```python
from build123d import *

# Parameters (mm, degrees)
RESSALTO_EXTRUS_O2_DEPTH      = 30
RESSALTO_EXTRUS_O3_START      = 3
RESSALTO_EXTRUS_O3_DEPTH      = 3
RESSALTO_EXTRUS_O4_DEPTH      = 3
RESSALTO_EXTRUS_O4_DEPTH_BACK = 10
CORTE_EXTRUS_O1_DEPTH         = 10.000000000000002
CORTE_EXTRUS_O2_REACH         = 83.702
FILETE1_R                     = 2


with BuildPart() as part:
    # Esboço2 → Ressalto-extrusão2 (new body)
    with BuildSketch(Plane(origin=(0, 0, 0), x_dir=(0, 0, -1), z_dir=(1, 0, 0))):
        with BuildLine():
            Line((2.901599919865161, -0.06246593766177921), (-35.09840008013481, -0.06246593766176534))
            Line((-35.09840008013481, -0.06246593766176534), (-39.886084902926825, -0.06246593766177921))
            ThreePointArc((-39.886084902926825, -0.06246593766177921), (-45.20218023363878, 1.4676385237390175), (-48.891439327799866, 5.589707975381692))
            ThreePointArc((-48.891439327799866, 5.589707975381692), (-52.09653694789475, 9.772081498832542), (-56.69840008013493, 12.338743680758546))
            ThreePointArc((-56.69840008013493, 12.338743680758546), (-59.37322401506481, 11.895603400997262), (-60.5984000801349, 9.476926076507686))
            Line((-60.5984000801349, 9.476926076507686), (-60.598400080134894, 20.976926076507663))
            ThreePointArc((-60.598400080134894, 20.976926076507663), (-59.71972042369454, 23.098246420067323), (-57.59840008013488, 23.976926076507684))
            Line((-57.59840008013488, 23.976926076507684), (25.401599919865156, 23.976926076507684))
            ThreePointArc((25.401599919865156, 23.976926076507684), (27.522920263424812, 23.098246420067333), (28.401599919865177, 20.976926076507684))
            Line((28.401599919865177, 20.976926076507684), (28.40159991986526, 9.476926076507686))
            ThreePointArc((28.40159991986526, 9.476926076507686), (27.176423854795164, 11.895603400997262), (24.50159991986529, 12.338743680758546))
            ThreePointArc((24.50159991986529, 12.338743680758546), (19.8997367876251, 9.772081498832549), (16.69463916753021, 5.589707975381692))
            ThreePointArc((16.69463916753021, 5.589707975381692), (13.005380073369123, 1.467638523739021), (7.689284742657176, -0.06246593766177921))
            Line((7.689284742657176, -0.06246593766177921), (2.901599919865161, -0.06246593766177921))
        make_face()
    extrude(amount=RESSALTO_EXTRUS_O2_DEPTH)

    # Esboço3 → Ressalto-extrusão3 (add)
    with BuildSketch(Plane.ZY.offset(RESSALTO_EXTRUS_O3_START)):
        with BuildLine():
            Line((60.598400080134894, 15.226926076507677), (60.59840008013489, 20.976926076507663))
            ThreePointArc((60.59840008013489, 20.976926076507663), (59.71972042369454, 23.098246420067326), (57.59840008013487, 23.976926076507684))
            Line((57.59840008013487, 23.976926076507684), (16.09840008013486, 23.976926076507684))
            Line((16.09840008013486, 23.976926076507684), (-25.4015999198652, 23.976926076507684))
            ThreePointArc((-25.4015999198652, 23.976926076507684), (-27.52292026342486, 23.098246420067326), (-28.40159991986522, 20.976926076507663))
            Line((-28.40159991986522, 20.976926076507663), (-28.40159991986522, 15.226926076507686))
            Line((-28.40159991986522, 15.226926076507686), (-28.40159991986525, -16.773073923492294))
            ThreePointArc((-28.40159991986525, -16.773073923492294), (-27.522920263424897, -18.894394267051958), (-25.401599919865234, -19.77307392349232))
            Line((-25.401599919865234, -19.77307392349232), (57.59840008013488, -19.773073923492326))
            ThreePointArc((57.59840008013488, -19.773073923492326), (59.71972042369455, -18.89439426705197), (60.5984000801349, -16.7730739234923))
            Line((60.5984000801349, -16.7730739234923), (60.598400080134894, 15.226926076507677))
        make_face()
    extrude(amount=-RESSALTO_EXTRUS_O3_DEPTH)

    # Esboço4 → Ressalto-extrusão4 (add, two sides: drawn at the far end of the back side and taken through both)
    with BuildSketch(Plane(origin=(30, 0, 0), x_dir=(0, 0, -1), z_dir=(1, 0, 0)).offset(-RESSALTO_EXTRUS_O4_DEPTH_BACK)):
        with BuildLine():
            Line((-16.09840008013486, 23.976926076507684), (25.4015999198652, 23.976926076507684))
            ThreePointArc((25.4015999198652, 23.976926076507684), (27.52292026342486, 23.098246420067326), (28.40159991986522, 20.976926076507663))
            Line((28.40159991986522, 20.976926076507663), (28.40159991986522, 15.226926076507686))
            Line((28.40159991986522, 15.226926076507686), (28.40159991986523, -16.773073923492294))
            ThreePointArc((28.40159991986523, -16.773073923492294), (27.522920263424872, -18.89439426705196), (25.401599919865205, -19.77307392349232))
            Line((25.401599919865205, -19.77307392349232), (-57.598400080134866, -19.773073923492326))
            ThreePointArc((-57.598400080134866, -19.773073923492326), (-59.71972042369453, -18.89439426705197), (-60.59840008013489, -16.773073923492305))
            Line((-60.59840008013489, -16.773073923492305), (-60.598400080134894, 15.226926076507677))
            Line((-60.598400080134894, 15.226926076507677), (-60.598400080134894, 20.976926076507663))
            ThreePointArc((-60.598400080134894, 20.976926076507663), (-59.71972042369454, 23.098246420067326), (-57.59840008013487, 23.976926076507684))
            Line((-57.59840008013487, 23.976926076507684), (-16.09840008013486, 23.976926076507684))
        make_face()
    extrude(amount=RESSALTO_EXTRUS_O4_DEPTH + RESSALTO_EXTRUS_O4_DEPTH_BACK)

    # Esboço8 → Corte-extrusão1 (cut)
    with BuildSketch(Plane(origin=(33, 0, 0), x_dir=(0, 0, -1), z_dir=(1, 0, 0))):
        with BuildLine():
            Line((-43.59840008013488, -2.7730739234923267), (11.401599919865212, -2.7730739234923267))
            ThreePointArc((11.401599919865212, -2.7730739234923267), (12.815813482238323, -3.3588603611192323), (13.401599919865227, -4.7730739234923405))
            Line((13.401599919865227, -4.7730739234923405), (13.401599919865227, -10.773073923492314))
            ThreePointArc((13.401599919865227, -10.773073923492314), (12.81581348223832, -12.187287485865422), (11.401599919865212, -12.773073923492326))
            Line((11.401599919865212, -12.773073923492326), (-43.59840008013488, -12.773073923492326))
            ThreePointArc((-43.59840008013488, -12.773073923492326), (-45.012613642507986, -12.187287485865422), (-45.598400080134894, -10.773073923492314))
            Line((-45.598400080134894, -10.773073923492314), (-45.598400080134894, -4.7730739234923405))
            ThreePointArc((-45.598400080134894, -4.7730739234923405), (-45.012613642507986, -3.358860361119232), (-43.59840008013488, -2.7730739234923267))
        make_face()
        with BuildLine():
            Line((-43.59840008013488, 6.976926076507685), (11.401599919865218, 6.976926076507685))
            ThreePointArc((11.401599919865218, 6.976926076507685), (12.815813482238326, 7.56271251413459), (13.401599919865228, 8.976926076507699))
            Line((13.401599919865228, 8.976926076507699), (13.401599919865227, 14.976926076507674))
            ThreePointArc((13.401599919865227, 14.976926076507674), (12.81581348223832, 16.39113963888078), (11.401599919865214, 16.976926076507684))
            Line((11.401599919865214, 16.976926076507684), (-43.59840008013488, 16.976926076507684))
            ThreePointArc((-43.59840008013488, 16.976926076507684), (-45.012613642507986, 16.39113963888078), (-45.598400080134894, 14.976926076507672))
            Line((-45.598400080134894, 14.976926076507672), (-45.598400080134894, 8.976926076507699))
            ThreePointArc((-45.598400080134894, 8.976926076507699), (-45.012613642507986, 7.5627125141345894), (-43.59840008013488, 6.976926076507685))
        make_face()
    extrude(amount=-CORTE_EXTRUS_O1_DEPTH, mode=Mode.SUBTRACT)

    # Esboço9 → Corte-extrusão2 (cut, up to next)
    with BuildSketch(Plane(origin=(0, -19.773073923492323, -1.65e-15), x_dir=(-1, 0, 0), z_dir=(0, -1, -8e-17)), mode=Mode.PRIVATE) as corte_extrus_o2_sk1:
        with BuildLine():
            Line((-25.000000000000007, 13.401599919865228), (-27.99999999999999, 13.401599919865228))
            ThreePointArc((-27.99999999999999, 13.401599919865228), (-29.414213562373096, 12.815813482238323), (-30.000000000000004, 11.401599919865216))
            Line((-30.000000000000004, 11.401599919865216), (-29.999999999999996, -43.59840008013487))
            ThreePointArc((-29.999999999999996, -43.59840008013487), (-29.414213562373092, -45.01261364250798), (-27.999999999999982, -45.59840008013489))
            Line((-27.999999999999982, -45.59840008013489), (-25, -45.59840008013489))
            ThreePointArc((-25, -45.59840008013489), (-23.585786437626894, -45.01261364250798), (-22.99999999999999, -43.59840008013487))
            Line((-22.99999999999999, -43.59840008013487), (-22.999999999999996, 11.401599919865216))
            ThreePointArc((-22.999999999999996, 11.401599919865216), (-23.585786437626897, 12.815813482238324), (-25.000000000000007, 13.401599919865228))
        make_face()
    corte_extrus_o2_tool1 = extrude(corte_extrus_o2_sk1.sketch, amount=-CORTE_EXTRUS_O2_REACH, mode=Mode.PRIVATE) & part.part
    add(corte_extrus_o2_tool1.solids().sort_by_distance((26.5, -19.773074, 16.0984))[0], mode=Mode.SUBTRACT)

    # Filete1
    # the kernel refuses this fillet: 2 mm, written as the material it adds along each edge
    with BuildSketch(Plane(origin=(22.99999999999999, -15.773073923492316, 45.59840008013489), x_dir=(0, 0, -1), z_dir=(0, 1, 0))) as filete1_piece_1:
        with BuildLine():
            CenterArc((FILETE1_R, -FILETE1_R), FILETE1_R, 90, 90)
            Line((0, -FILETE1_R), (0, 0))
            Line((0, 0), (FILETE1_R, 0))
        make_face()
    extrude(amount=10.999999999999973)
    with BuildSketch(Plane(origin=(23, -4.773073923492332, 43.59840008013489), x_dir=(0, -4.44e-15, 1), z_dir=(0, -1, -4.44e-15))) as filete1_piece_2:
        with BuildLine():
            CenterArc((2.000000000000007 - FILETE1_R, -FILETE1_R), FILETE1_R, 359.9999999999997, 90.00000000000028)
            Line((2.000000000000007, -FILETE1_R), (2.000000000000007, 0))
            Line((2.000000000000007, 0), (2.000000000000007 - FILETE1_R, 1.066e-14))
        make_face()
    revolve(axis=Axis((23, -4.773073923492332, 43.59840008013489), (-1, 0, 0)), revolution_arc=90.00000000000045)
    with BuildSketch(Plane(origin=(23, -2.7730739234923267, 43.59840008013488), x_dir=(-5.33e-15, -1, 0), z_dir=(0, 0, -1))) as filete1_piece_3:
        with BuildLine():
            CenterArc((FILETE1_R, -FILETE1_R), FILETE1_R, 89.99999999999969, 90.00000000000031)
            Line((-1.11e-14, -FILETE1_R), (0, 0))
            Line((0, 0), (FILETE1_R, 0))
        make_face()
    extrude(amount=55.00000000000009)
    with BuildSketch(Plane(origin=(23, -4.773073923492328, -11.401599919865227), x_dir=(0, 1, 7.11e-15), z_dir=(0, -7.11e-15, 1))) as filete1_piece_4:
        with BuildLine():
            CenterArc((2.0000000000000004 - FILETE1_R, -FILETE1_R), FILETE1_R, 359.9999999999999, 90.00000000000011)
            Line((2.0000000000000018, -FILETE1_R), (2.0000000000000004, 0))
            Line((2.0000000000000004, 0), (2.0000000000000004 - FILETE1_R, 3.55e-15))
        make_face()
    revolve(axis=Axis((23, -4.773073923492328, -11.401599919865227), (-1, 0, 0)), revolution_arc=90.00000000000077)
    with BuildSketch(Plane(origin=(23, -4.7730739234923405, -13.401599919865227), x_dir=(-1.78e-15, 0, 1), z_dir=(0, -1, 0))) as filete1_piece_5:
        with BuildLine():
            CenterArc((FILETE1_R, -FILETE1_R), FILETE1_R, 89.9999999999999, 90.0000000000001)
            Line((-3.55e-15, -FILETE1_R), (0, 0))
            Line((0, 0), (FILETE1_R, 0))
        make_face()
    extrude(amount=10.999999999999973)


solid = part.part
```
Work out the finished part from the listing and answer in its coordinate system (mm). A direction names the side the tool comes from. Give positions to 0.01 mm unless a question says otherwise; leave off trailing zeros. Loops run counter-clockwise (first coordinate to the right, second up) from the corner with the lowest first, then second, coordinate; pieces in that order, holes last. Notation, with made-up numbers: (-16.5, 1) -> (-12.5, 1) arc R9 ccw to (-12.5, 9) -> close; hole circle Ø3 at (39, -26). An arc over 180 degrees is marked (long way). Write item = value, one per line. Start each with the question number.
(1) Given pin 1 Ø11 at (x, z) = (29.5, 15.5) entering from -Y; pin 2 Ø2.5 at (x, z) = (27.5, 21.5) entering from -Y; pin 3 Ø3 at (y, z) = (11.5, 11.5) entering from +X, each flat-ended and moving along its own axis, determine where each tip first touches the part or whether it passes through.
(2) Find the intervals of material crossed by probe 1 along X at (y, z) = (-17, 12.5); probe 2 along X at (y, z) = (-7, 26); probe 3 along X at (y, z) = (-4, -21), in increasing order. Write a range as from..to.
(3) Find section C-C on z = 30.5. Give the vertices of the cut face in (x, y), and give its area (3 significant figures).
(4) Find section D-D on x = 16. Give the vertices of the cut face in (y, z), and give its area (3 significant figures).
(5) Find section A-A on y = -15. Give the vertices of the cut face in (x, z).
(6) The mould has two halves that part along X. Classify faces 3 (the flat face through (32, -12.773, 16)), 4 (the cylindrical face through (23.57, -3.374, 16.483)), 5 (the flat face through (27, -11, 45.598)): +X half, -X half, draft (parallel to the pull), parting line (faces both ways), or undercut.
(7) Find section B-B on y = -1. Give the vertices of the cut face in (x, z).
(8) Which of the six approach directions +Z, -Z, +X, -X, +Y, -Y give full straight-line access (tool end or side, diameter ignored) to faces 1 (the cylindrical face through (31.091, -12.172, -12.831)), 2 (the cylindrical face through (-1.521, -18.871, -27.546))?
From the geometry:
q1.pin_1 = -19.77
q1.pin_2 = -2.77
q1.pin_3 = 23
q2.probe_1 = -3..0, 20..23, 30..33
q2.probe_2 = -3..0, 20..23
q2.probe_3 = -3..0, 20..33
q3.outline = (-3, -19.77) -> (0, -19.77) -> (0, -0.06) -> (20, -0.06) -> (20, -19.77) -> (23, -19.77) -> (23, -4.77) arc R2 cw to (25, -2.77) -> (33, -2.77) -> (33, 6.98) -> (23, 6.98) -> (23, 16.98) -> (33, 16.98) -> (33, 23.98) -> (-3, 23.98) -> close; (30, -19.77) -> (33, -19.77) -> (33, -12.77) -> (30, -12.77) -> close
q3.area = 933 mm^2
q4.outline = (-0.06, -7.69) arc R10 ccw to (5.59, -16.69) arc R13 cw to (12.34, -24.5) arc R3 cw to (9.48, -28.4) -> (20.98, -28.4) arc R3 ccw to (23.98, -25.4) -> (23.98, 57.6) arc R3 ccw to (20.98, 60.6) -> (9.48, 60.6) arc R3 cw to (12.34, 56.7) arc R13 cw to (5.59, 48.89) arc R10 ccw to (-0.06, 39.89) -> close
q4.area = 1,860 mm^2
q5.outline = (-3, -28.4) -> (0, -28.4) -> (0, 60.6) -> (-3, 60.6) -> close; (20, -28.4) -> (33, -28.4) -> (33, 60.6) -> (20, 60.6) -> close; hole (23, -11.4) arc R2 ccw to (25, -13.4) -> (28, -13.4) arc R2 ccw to (30, -11.4) -> (30, 43.6) arc R2 ccw to (28, 45.6) -> (25, 45.6) arc R2 ccw to (23, 43.6) -> close
q6.face_3 = draft
q6.face_4 = +X half
q6.face_5 = undercut
q7.outline = (-3, -28.4) -> (0, -28.4) -> (0, 60.6) -> (-3, 60.6) -> close; (20, -28.4) -> (33, -28.4) -> (33, 60.6) -> (20, 60.6) -> close
q8.face_1 = +X
q8.face_2 = -Z, +X, -X, -Y
